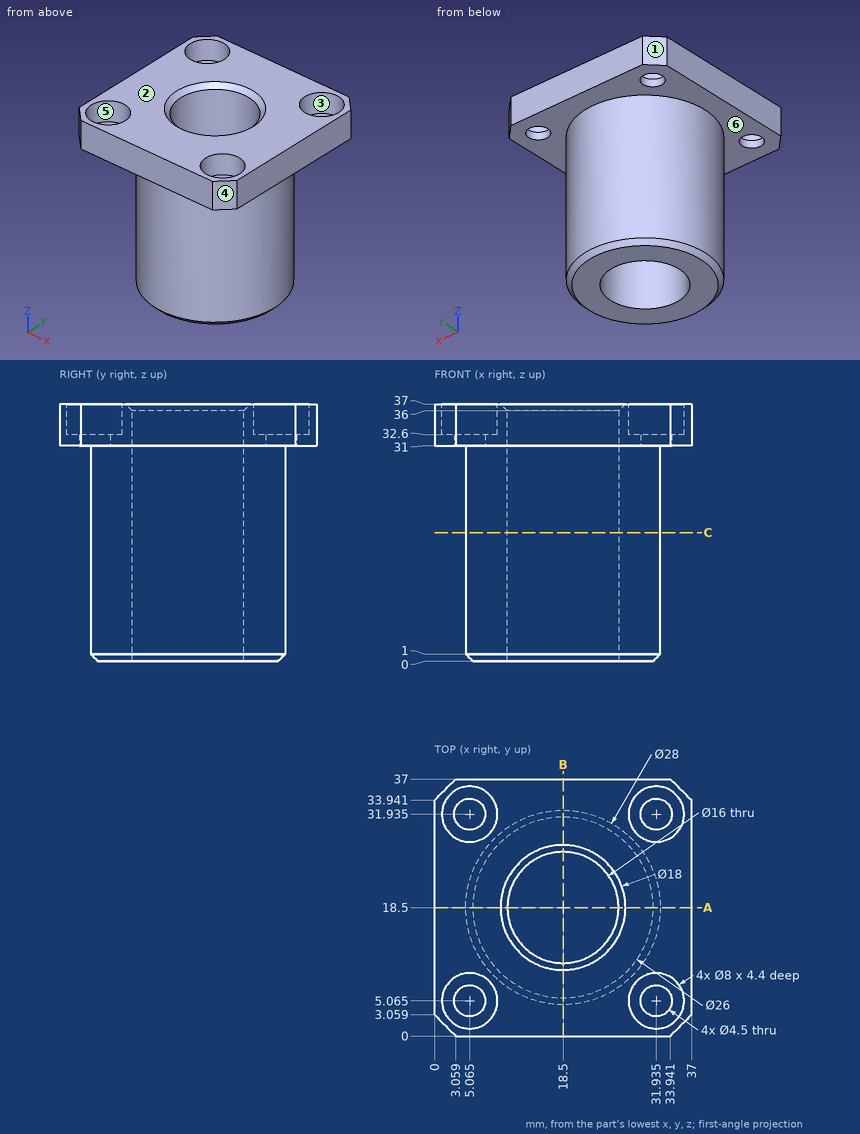
Job drawing, mm, ordinate dimensions from the low corner. One solid piece. A direction names the side the tool comes from. Give positions to 0.01 mm unless a question says otherwise; leave off trailing zeros. Write each loop counter-clockwise with the first axis right and the second up, starting at its lowest first coordinate (ties: lowest second). Pieces come first, ordered by that corner, then holes. Notation, with made-up numbers: M 20.25,72 L 31.25,72 A20 cw 31.25,80 Z; hole C 17,72 d1. An arc over 180 degrees is marked long. Put each result on its own line as item: value. Start each with the question number.
(1) Probe L1, parallel to Y at x = 33, z = 34.5; L2, parallel to Y at x = 6.5, z = 33.5; L3, parallel to X at y = 17, z = 32. List the from-to ranges inside material, lowest first.
(2) Mould opens along X. For the marked faces 1, 2 and 3 say: +X half, -X half, draft (parallel to the pull), parting line (faces both ways), or undercut.
(3) Flat gauge pins, fed straight in: pin 1 Ø4 at (x, y) = (4, 34) entering from +Z; pin 2 Ø5 at (x, z) = (28, 9) entering from -Y; pin 3 Ø7 at (x, y) = (31.94, 31.94) entering from +Z; pin 4 Ø5 at (x, y) = (31.94, 31.94) entering from -Z. Where does each tip first touch, or does it go through?
(4) Band-saw the part on A-A, the plane y = 18.5. Write the cut outline in (x, z), and give its area (3 significant figures).
(5) Which spindle directions (+Z, -Z, +X, -X, +Y, -Y) get a long thin tool onto all of the face, cutting with end or side? Do the marked faces 4, 5 and 6. Say none if no direction does.
(6) Band-saw the part on C-C, the plane z = 18.5. Write the cut outline in (x, y), and give its area (3 significant figures).
Response values:
1. L1: y = 0 to 1.21, 8.92 to 28.08, 35.79 to 37
1. L2: y = 0 to 1.33, 8.8 to 28.2, 35.67 to 37
1. L3: x = 0 to 10.64, 26.36 to 37
2. face 1: -X half
2. face 2: draft
2. face 3: undercut
3. pin 1: stops at z = 37
3. pin 2: stops at y = 6.38
3. pin 3: stops at z = 32.6
3. pin 4: stops at z = 31
4. outline: M 0,31 L 4.5,31 L 4.5,1 L 5.5,0 L 10.5,0 L 10.5,36 L 9.5,37 L 0,37 Z; M 26.5,0 L 31.5,0 L 32.5,1 L 32.5,31 L 37,31 L 37,37 L 27.5,37 L 26.5,36 Z
4. area: 496 mm2
5. face 4: +Z, -Z, +X, -Y
5. face 5: +Z
5. face 6: -Z
6. outline: C 18.5,18.5 d28; hole C 18.5,18.5 d16
6. area: 415 mm2
